from build123d import *

# Parameters (mm, degrees)
ESQUISSE1_R                                  = 32.5
BOSS_EXTRU_1_DEPTH                           = 5
ESQUISSE2_R                                  = 22.5
ENL_V_MAT_EXTRU_1_DEPTH                      = 2.5
ESQUISSE3_R                                  = 6.5
ENL_V_MAT_EXTRU_2_DEPTH                      = 47.029881599
TROUS_DE_CENTRAGE_6_0MM1_D                   = 6
ESQUISSE6_W                                  = 105
ESQUISSE6_H                                  = 74
ESQUISSE6_R                                  = 32.5
BOSS_EXTRU_2_DEPTH                           = 10
ESQUISSE7_R                                  = 32.5
ESQUISSE7_R_2                                = 3
ESQUISSE7_R_3                                = 22.5
BOSS_EXTRU_3_DEPTH                           = 10.5
CHAMBRAGE_POUR_VIS_T_TE_RONDE_BOMB_2_COUNT   = 2
CHAMBRAGE_POUR_VIS_T_TE_RONDE_BOMB_2_PITCH   = 43.634433716
CHAMBRAGE_POUR_VIS_T_TE_RONDE_BOMB_3_COUNT   = 2
CHAMBRAGE_POUR_VIS_T_TE_RONDE_BOMB_3_PITCH   = 43.634433716
ESQUISSE16_R                                 = 6.5
BOSS_EXTRU_4_DEPTH                           = 8
CHAMBRAGE_POUR_VIS_T_TE_RONDE_BOMB_5_A_COUNT = 2
CHAMBRAGE_POUR_VIS_T_TE_RONDE_BOMB_5_A_PITCH = 43.634433716
D_GAGEMENT_M33_D                             = 3.4
D_GAGEMENT_M33_DEPTH                         = 5
D_GAGEMENT_M33_TIP                           = 0.981495458
D_GAGEMENT_M42_D                             = 4.5
D_GAGEMENT_M42_DEPTH                         = 5
D_GAGEMENT_M42_TIP                           = 1.299038106
D_GAGEMENT_M43_D                             = 4.5
D_GAGEMENT_M43_DEPTH                         = 5
D_GAGEMENT_M43_TIP                           = 1.299038106
D_GAGEMENT_M44_D                             = 4.5
D_GAGEMENT_M44_DEPTH                         = 5
D_GAGEMENT_M44_TIP                           = 1.299038106
D_GAGEMENT_M45_D                             = 4.5
D_GAGEMENT_M45_DEPTH                         = 3
D_GAGEMENT_M45_TIP                           = 1.299038106


with BuildPart() as part:
    # Esquisse1 → Boss.-Extru.1 (new body)
    with BuildSketch(Plane.XY):
        Circle(ESQUISSE1_R)
    extrude(amount=BOSS_EXTRU_1_DEPTH)

    # Esquisse2 → Enlèv. mat.-Extru.1 (cut)
    with BuildSketch(Plane.XY.offset(5)):
        Circle(ESQUISSE2_R)
    extrude(amount=-ENL_V_MAT_EXTRU_1_DEPTH, mode=Mode.SUBTRACT)

    # Esquisse3 → Enlèv. mat.-Extru.2 (cut, through all)
    with BuildSketch(Plane.XY.offset(2.5)):
        Circle(ESQUISSE3_R)
    extrude(amount=-ENL_V_MAT_EXTRU_2_DEPTH, mode=Mode.SUBTRACT)

    # Trous de centrage Ø6.0mm1 (through all)
    with Locations(Plane.XY.offset(5)):
        with Locations((0, -27.5), (-26.562960223, 7.11752374), (26.562960223, 7.11752374)):
            Hole(TROUS_DE_CENTRAGE_6_0MM1_D / 2)

    # Esquisse6 → Boss.-Extru.2 (add)
    with BuildSketch(Plane(origin=(0, 0, 0), x_dir=(-1, 0, 0), z_dir=(0, 0, -1))):
        with Locations((17.555230344, -3.167731133)):
            Rectangle(ESQUISSE6_W, ESQUISSE6_H)
        Circle(ESQUISSE6_R, mode=Mode.SUBTRACT)
    extrude(amount=-BOSS_EXTRU_2_DEPTH)

    # Esquisse7 → Boss.-Extru.3 (add)
    with BuildSketch(Plane.XY.offset(5)):
        with Locations(Location((0, 0, 0), (0, 0, 180))):
            Circle(ESQUISSE7_R)
        with Locations((0, -27.5)):
            Circle(ESQUISSE7_R_2, mode=Mode.SUBTRACT)
        with Locations((-26.562960223, 7.11752374)):
            Circle(ESQUISSE7_R_2, mode=Mode.SUBTRACT)
        Circle(ESQUISSE7_R_3, mode=Mode.SUBTRACT)
        with Locations((26.562960223, 7.11752374)):
            Circle(ESQUISSE7_R_2, mode=Mode.SUBTRACT)
    extrude(amount=BOSS_EXTRU_3_DEPTH)

    # Esquisse14 → Chambrage pour vis _ t_te ronde bomb_e M (revolve, cut)
    with BuildSketch(Plane(origin=(0, -27.5, 0), x_dir=(0, 1, 0), z_dir=(1, 0, 0))):
        Polygon((0, 0), (0, 6.982840043), (3.3, 5), (3.3, 4.625), (3.325, 4.6), (6.5, 4.6), (6.5, 0), align=None)
    chambrage_pour_vis_t_te_ronde_bomb_e_m = revolve(axis=Axis((0, -27.5, -6.35), (0, 0, 1)), mode=Mode.SUBTRACT)

    # Chambrage pour vis _ t_te ronde bomb 2: Chambrage pour vis _ t_te ronde bomb_e M ×2
    with Locations(*[Vector(-0.6087614290087126, 0.7933533402912415, 0) * (i * CHAMBRAGE_POUR_VIS_T_TE_RONDE_BOMB_2_PITCH) for i in range(1, CHAMBRAGE_POUR_VIS_T_TE_RONDE_BOMB_2_COUNT)]):
        add(chambrage_pour_vis_t_te_ronde_bomb_e_m, mode=Mode.SUBTRACT)

    # Chambrage pour vis _ t_te ronde bomb 3: Chambrage pour vis _ t_te ronde bomb_e M ×2
    with Locations(*[Vector(0.6087614290087182, 0.793353340291237, 0) * (i * CHAMBRAGE_POUR_VIS_T_TE_RONDE_BOMB_3_PITCH) for i in range(1, CHAMBRAGE_POUR_VIS_T_TE_RONDE_BOMB_3_COUNT)]):
        add(chambrage_pour_vis_t_te_ronde_bomb_e_m, mode=Mode.SUBTRACT)

    # Esquisse16 → Boss.-Extru.4 (add)
    # profile 1 of 4: a face of its own
    with BuildSketch(Plane.XY.offset(2.5)):
        with BuildLine():
            ThreePointArc((-22.399321758, 2.126119656), (-17.850450157, -13.697132153), (-3.743697183, -22.186363636))
            ThreePointArc((-3.743697183, -22.186363636), (0, -21), (3.743697183, -22.186363636))
            ThreePointArc((3.743697183, -22.186363636), (17.850450157, -13.697132153), (22.399321758, 2.126119656))
            ThreePointArc((22.399321758, 2.126119656), (20.284442352, 5.435199947), (20.461441498, 9.358387245))
            ThreePointArc((20.461441498, 9.358387245), (0, 22.5), (-20.461441498, 9.358387245))
            ThreePointArc((-20.461441498, 9.358387245), (-20.284442352, 5.435199947), (-22.399321758, 2.126119656))
        make_face()
        Circle(ESQUISSE16_R, mode=Mode.SUBTRACT)
    # profile 2 of 4: a face of its own
    with BuildSketch(Plane.XY.offset(2.5)):
        with BuildLine():
            ThreePointArc((20.461441498, 9.358387245), (20.284442352, 5.435199947), (22.399321758, 2.126119656))
            ThreePointArc((22.399321758, 2.126119656), (21.733331092, 5.823428515), (20.461441498, 9.358387245))
        make_face()
    # profile 3 of 4: a face of its own
    with BuildSketch(Plane.XY.offset(2.5)):
        with BuildLine():
            ThreePointArc((-3.743697183, -22.186363636), (0, -22.5), (3.743697183, -22.186363636))
            ThreePointArc((3.743697183, -22.186363636), (0, -21), (-3.743697183, -22.186363636))
        make_face()
    # profile 4 of 4: a face of its own
    with BuildSketch(Plane.XY.offset(2.5)):
        with BuildLine():
            ThreePointArc((-22.399321758, 2.126119656), (-20.284442352, 5.435199947), (-20.461441498, 9.358387245))
            ThreePointArc((-20.461441498, 9.358387245), (-21.733331092, 5.823428515), (-22.399321758, 2.126119656))
        make_face()
    extrude(amount=BOSS_EXTRU_4_DEPTH)

    # Esquisse17 → Chambrage pour vis _ t_te ronde bomb 4 (revolve, cut)
    with BuildSketch(Plane(origin=(-26.562960223, 7.11752374, 0), x_dir=(0, 1, 0), z_dir=(1, 0, 0))):
        Polygon((0, 0), (0, 6.982840043), (3.3, 5), (3.3, 4.625), (3.325, 4.6), (6.5, 4.6), (6.5, 0), align=None)
    revolve(axis=Axis((-26.562960223, 7.11752374, -6.35), (0, 0, 1)), mode=Mode.SUBTRACT)

    # Esquisse19 → Chambrage pour vis _ t_te ronde bomb 5 (revolve, cut)
    with BuildSketch(Plane(origin=(0, -27.5, 0), x_dir=(0, 1, 0), z_dir=(1, 0, 0))):
        Polygon((0, 0), (0, 6.982840043), (3.3, 5), (3.3, 4.625), (3.325, 4.6), (6.5, 4.6), (6.5, 0), align=None)
    chambrage_pour_vis_t_te_ronde_bomb_5 = revolve(axis=Axis((0, -27.5, -6.35), (0, 0, 1)), mode=Mode.SUBTRACT)

    # Chambrage pour vis _ t_te ronde bomb 5 a: Chambrage pour vis _ t_te ronde bomb 5 ×2
    with Locations(*[Vector(0.6087614290087182, 0.793353340291237, 0) * (i * CHAMBRAGE_POUR_VIS_T_TE_RONDE_BOMB_5_A_PITCH) for i in range(1, CHAMBRAGE_POUR_VIS_T_TE_RONDE_BOMB_5_A_COUNT)]):
        add(chambrage_pour_vis_t_te_ronde_bomb_5, mode=Mode.SUBTRACT)

    # Dégagement M33
    with Locations(Plane(origin=(0, 0, 0), x_dir=(-1, 0, 0), z_dir=(0, 0, -1))):
        with Locations((55.547535515, -22.294087775), (36.229018989, -17.117706873), (55.547535515, 22.294087775), (36.229018989, 17.117706873), (38.2648555, 10.872157738), (30.699885045, 25.058257509), (37.238947698, 26.810394066), (38.2648555, -10.872157738), (37.238947698, -26.810394066), (30.699885045, -25.058257509), (62.293797593, 3.775), (62.293797593, -3.775)):
            Hole(D_GAGEMENT_M33_D / 2, depth=D_GAGEMENT_M33_DEPTH)
            with Locations((0, 0, -(D_GAGEMENT_M33_DEPTH + D_GAGEMENT_M33_TIP / 2))):  # 120° drill point
                Cone(0, D_GAGEMENT_M33_D / 2, D_GAGEMENT_M33_TIP, mode=Mode.SUBTRACT)

    # Dégagement M42
    with Locations(Plane(origin=(0, 0, 0), x_dir=(-1, 0, 0), z_dir=(0, 0, -1))):
        with Locations((38.293797593, 0)):
            Hole(D_GAGEMENT_M42_D / 2, depth=D_GAGEMENT_M42_DEPTH)
            with Locations((0, 0, -(D_GAGEMENT_M42_DEPTH + D_GAGEMENT_M42_TIP / 2))):  # 120° drill point
                Cone(0, D_GAGEMENT_M42_D / 2, D_GAGEMENT_M42_TIP, mode=Mode.SUBTRACT)

    # Dégagement M43
    with Locations(Plane(origin=(0, 0, 0), x_dir=(-1, 0, 0), z_dir=(0, 0, -1))):
        with Locations((62.420130644, 28.906134766)):
            Hole(D_GAGEMENT_M43_D / 2, depth=D_GAGEMENT_M43_DEPTH)
            with Locations((0, 0, -(D_GAGEMENT_M43_DEPTH + D_GAGEMENT_M43_TIP / 2))):  # 120° drill point
                Cone(0, D_GAGEMENT_M43_D / 2, D_GAGEMENT_M43_TIP, mode=Mode.SUBTRACT)

    # Dégagement M44
    with Locations(Plane(origin=(0, 0, 0), x_dir=(-1, 0, 0), z_dir=(0, 0, -1))):
        with Locations((61.930509464, -28.264433855)):
            Hole(D_GAGEMENT_M44_D / 2, depth=D_GAGEMENT_M44_DEPTH)
            with Locations((0, 0, -(D_GAGEMENT_M44_DEPTH + D_GAGEMENT_M44_TIP / 2))):  # 120° drill point
                Cone(0, D_GAGEMENT_M44_D / 2, D_GAGEMENT_M44_TIP, mode=Mode.SUBTRACT)

    # Dégagement M45
    with Locations(Plane(origin=(0, 0, 0), x_dir=(-1, 0, 0), z_dir=(0, 0, -1))):
        with Locations((23.628478868, -35.912807339), (23.628478868, 29.577345073), (-29.371521132, 29.577345073), (-29.371521132, -35.912807339)):
            Hole(D_GAGEMENT_M45_D / 2, depth=D_GAGEMENT_M45_DEPTH)
            with Locations((0, 0, -(D_GAGEMENT_M45_DEPTH + D_GAGEMENT_M45_TIP / 2))):  # 120° drill point
                Cone(0, D_GAGEMENT_M45_D / 2, D_GAGEMENT_M45_TIP, mode=Mode.SUBTRACT)


solid = part.part
Verification items for the finished model (mm, model axes). A direction names the side the tool comes from. Give positions to 0.01 mm unless a question says otherwise; leave off trailing zeros. Write each loop counter-clockwise with the first axis right and the second up, starting at its lowest first coordinate (ties: lowest second). Pieces come first, ordered by that corner, then holes. Notation, with made-up numbers: M -38,77 L -25,77 A12 ccw -25,88 Z; hole C 68.25,75 d4. An arc over 180 degrees is marked long. Use CSV: the item, a comma, the result in double quotes.
1) Cross-section at B-B (x = -15.5). Enter the section's corners in (y, z), plus the area to 3 significant figures.
Final values:
outline,"M -40.17,0 L 33.83,0 L 33.83,10 L 28.57,10 L 28.57,15.5 L 16.31,15.5 L 16.31,10.5 L -16.31,10.5 L -16.31,15.5 L -28.57,15.5 L -28.57,10 L -40.17,10 Z"
area,"891 mm²"
2) Cross-section at C-C (x = -52.5). Enter the section's corners in (y, z), plus the area to 3 significant figures.
Final values:
outline,"M -40.17,0 L 33.83,0 L 33.83,10 L -40.17,10 Z"
area,"740 mm²"
3) Material ranges on line 1 along Y through (x, z) = (0, 4.75); line 2 along Y through (x, z) = (-26.5, 8); line 3 along X through (y, z) = (-4, 3), recorded low to high.
Final values:
line 1,"-40.17 to -30.8, -24.2 to -6.5, 6.5 to 33.83"
line 2,"-40.17 to 4.12, 10.12 to 33.83"
line 3,"-70.06 to -63.98, -60.61 to -5.12, 5.12 to 34.94"
4) Access from +Z, -Z, +X, -X, +Y, -Y to the whole of each face (thin tool, end or side, straight path). Record for faces 5 (the face through (-17, 33.832, 5)), 6 (the face through (30.41, -37.91, 1.52)).
Final values:
face 5,"+Z, -Z, +X, -X, +Y"
face 6,"-Z"
5) Cross-section at A-A (z = 13.75). Enter the section's corners in (x, y), plus the area to 3 significant figures.
Final values:
outline,"C 0,0 d65; hole C -26.56,7.12 d6; hole C 0,0 d45; hole C 0,-27.5 d6; hole C 26.56,7.12 d6"
area,"1,640 mm²"
6) Go/stop test with flat-tipped pins: pin 1 Ø2.5 at (x, y) = (-23.63, 29.58) entering from +Z; pin 2 Ø2 at (x, y) = (-36.23, 17.12) entering from -Z; pin 3 Ø8.5 at (x, y) = (26.56, 7.12) entering from -Z. Record where each tip stops, or that it passes through.
Final values:
pin 1,"z = 10"
pin 2,"z = 5.4"
pin 3,"z = 4.6"
7) Release check for a two-part mould opening along X. For faces 1 (the face through (-70.055, -4, 5)), 2 (the face through (-37.9, 0.02, 6.07)), 3 (the face through (34.945, -4, 5)), 4 (the face through (-38.937, -26.736, 2.535)) record: released by +X, released by -X, zero draft, split by the parting line, or undercut.
Final values:
face 1,"released by -X"
face 2,"undercut"
face 3,"released by +X"
face 4,"undercut"
8) Cross-section at D-D (x = 13.5). Enter the section's corners in (y, z).
Final values:
outline,"M -40.17,0 L 33.83,0 L 33.83,10 L 29.56,10 L 29.56,15.5 L 18,15.5 L 18,10.5 L -18,10.5 L -18,15.5 L -29.56,15.5 L -29.56,10 L -40.17,10 Z"
